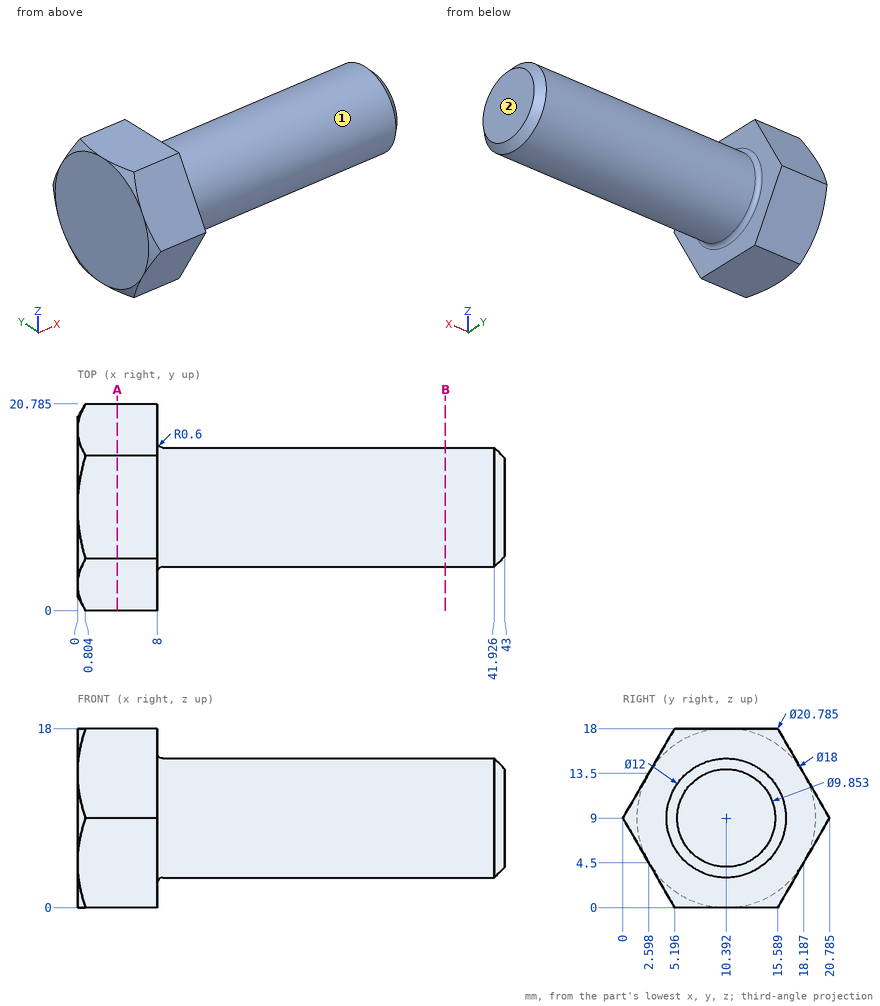
Here's the drawing with two shaded views (mm, measured from the low corner). I have some questions. A direction names the side the tool comes from. Coordinates: 2 decimals unless noted, no trailing zeros. Write each loop counter-clockwise with the first axis right and the second up, starting at its lowest first coordinate (ties: lowest second). Pieces come first, ordered by that corner, then holes. Notation, with made-up numbers: M 87,-15 L 128,-15 A14 ccw 128,1 Z; hole C 17.25,-37.5 d9. An arc over 180 degrees is marked long. Answer as CSV lines item,"result". Start each with the question number.
1) For the marked faces 1 and 2, which set-ups out of +Z, -Z, +X, -X, +Y, -Y let a thin tool reach every point of the face, with its end or its side?
2) For P1, Ø6, axis at x = 38, z = 3, coming from the -Y side (1 decimal); P2, Ø2, axis at x = 33.5, z = 10.5, coming from the -Y side; P3, Ø12, axis at x = 15, y = 8, coming from the -Z side, each with a flat end and sliding along its axis, tell me the tip position at first contact or that it passes through.
3) Please list where these lines run through material, in increasing order: line 1 (Y direction, x = 12, z = 12) (1 decimal); line 2 (X direction, y = 18, z = 6); line 3 (Z direction, x = 40, y = 5.5) (1 decimal). Write a range as from..to.
4) I want a section at B-B, the plane x = 37. Please give me the cut outline in (y, z).
5) I want a section at A-A, the plane x = 4. Please give me the cut outline in (y, z) (1 decimal), and give its area (3 significant figures).
Data:
1,face 1,"+X"
1,face 2,"+Z, -Z, +X, +Y, -Y"
2,P1,"stops at y = 5.2"
2,P2,"stops at y = 4.41"
2,P3,"stops at z = 3"
3,line 1,"y = 5.2..15.6"
3,line 2,"x = 0..8"
3,line 3,"z = 5.5..12.5"
4,outline,"C 10.39,9 d12"
5,outline,"M 0,9 L 5.2,0 L 15.6,0 L 20.8,9 L 15.6,18 L 5.2,18 Z"
5,area,"281 mm^2"
